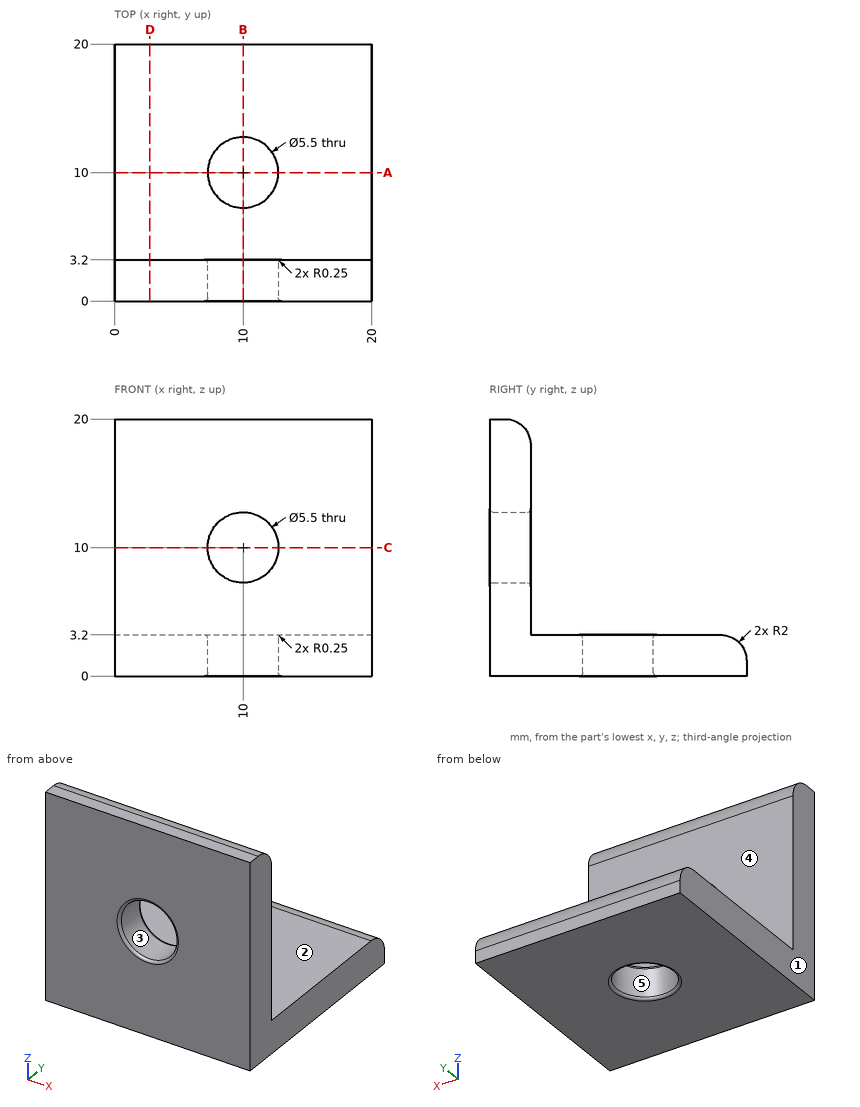
Geometry: see drawing. Coordinates: mm, zero at the bounding-box minimum. A direction names the side the tool comes from. Coordinates: 2 decimals unless noted, no trailing zeros. Order: outer loops, then holes, each group sorted by start corner. A loop starts at its lowest first (then second) coordinate and runs counter-clockwise, first axis right, second up. Notation, with made-up numbers: (45, 84.25) -> (100, 84.25) arc R14 cw to (100, 99.25) -> close; hole circle Ø9 at (25.5, -8). An arc over 180 degrees is marked (long way). Write each question's results on one line, items separated by ' | '. Start each with the question number.
1) First-contact query: pin 1 (12 mm diameter, centred on x = 15, z = 14, fed in from +Y); pin 2 (6 mm diameter, centred on x = 13.5, y = 8.5, fed in from +Z). Flat tips, straight axial feed; report the tip coordinate or a pass-through.
2) Set-up query: the marked faces 4 and 5. Return all of +Z, -Z, +X, -X, +Y, -Y with unobstructed straight access to the full face (end or side cutting, diameter ignored); none if empty.
3) Mould query, pull axis Z, two halves, no side actions, for the marked faces 1, 2 and 3. Classes: released by +Z, released by -Z, zero draft, split by the parting line, or undercut.
4) Material intervals for line 1 along X through (y, z) = (1.1, 10), sorted ascending.
5) Cut plane A-A, the plane y = 10. Output: boundary loops of the cut face in (x, z).
6) Cut plane B-B, the plane x = 10. Output: boundary loops of the cut face in (y, z), and give its area (3 significant figures).
7) Cut plane D-D, the plane x = 2.75. Output: boundary loops of the cut face in (y, z), and give its area (3 significant figures).
Checks:
1) pin 1: y = 3.2 | pin 2: z = 3.2
2) face 4: +Z, +X, -X, +Y | face 5: +Z, -Z
3) face 1: zero draft | face 2: released by +Z | face 3: undercut
4) line 1: 0 to 7.25, 12.75 to 20
5) outline: (0, 0) -> (7, 0) arc R0.25 ccw to (7.25, 0.25) -> (7.25, 2.95) arc R0.25 ccw to (7, 3.2) -> (0, 3.2) -> close; (12.75, 0.25) arc R0.25 ccw to (13, 0) -> (20, 0) -> (20, 3.2) -> (13, 3.2) arc R0.25 ccw to (12.75, 2.95) -> close
6) outline: (0, 0) -> (7, 0) arc R0.25 ccw to (7.25, 0.25) -> (7.25, 2.95) arc R0.25 ccw to (7, 3.2) -> (3.2, 3.2) -> (3.2, 7) arc R0.25 ccw to (2.95, 7.25) -> (0.25, 7.25) arc R0.25 ccw to (0, 7) -> close; (0, 13) arc R0.25 ccw to (0.25, 12.75) -> (2.95, 12.75) arc R0.25 ccw to (3.2, 13) -> (3.2, 18) arc R2 ccw to (1.2, 20) -> (0, 20) -> close; (12.75, 0.25) arc R0.25 ccw to (13, 0) -> (20, 0) -> (20, 1.2) arc R2 ccw to (18, 3.2) -> (13, 3.2) arc R0.25 ccw to (12.75, 2.95) -> close | area: 80.7 mm^2
7) outline: (0, 0) -> (20, 0) -> (20, 1.2) arc R2 ccw to (18, 3.2) -> (3.2, 3.2) -> (3.2, 18) arc R2 ccw to (1.2, 20) -> (0, 20) -> close | area: 116 mm^2
